Verification items for the finished model (mm, model axes). A direction names the side the tool comes from. Give positions to 0.01 mm unless a question says otherwise; leave off trailing zeros. Write each loop counter-clockwise with the first axis right and the second up, starting at its lowest first coordinate (ties: lowest second). Pieces come first, ordered by that corner, then holes. Notation, with made-up numbers: (-11.5, 9) -> (37.5, 9) arc R23 ccw to (37.5, 27) -> close; hole circle Ø2 at (77.5, 70.5). An arc over 180 degrees is marked (long way). Use one line per item in the form item = value. Start each with the question number.
(1) Section check D-D, the plane y = 6. Record the cut outline in (x, z).
(2) Section check A-A, the plane x = 0.5. Record the cut outline in (y, z).
(3) Set-up check for faces 4 (the face through (-61.486, 1, -29)), 5 (the face through (-23, 2.5, 14)), 6 (the face through (-63.486, 27, 26)), 7 (the face through (-17.486, 1, 26)): record each of +Z, -Z, +X, -X, +Y, -Y from which the full face is reachable in a straight line by a thin tool's end or side.
(4) Section check C-C, the plane z = -5. Record the cut outline in (x, y), plus the area to 3 significant figures.
(5) Scan lines: L1, parallel to X at y = 5.5, z = 20.5; L2, parallel to Z at x = 31, y = 7.25; L3, parallel to Y at x = -4.5, z = 20. Record each from-to range of solid material in increasing order.
(6) Section check B-B, the plane y = 20. State how many separate pieces and enclosed holes the cut face has, plus the area to 4 significant figures.
(7) Depth check by flat-ended pin: pin 1 Ø9.5 at (x, z) = (-23.49, -16.85) entering from +Y; pin 2 Ø1.5 at (y, z) = (28, 25.5) entering from +X; pin 3 Ø3.5 at (y, z) = (16, -29.5) entering from +X. Enter the tip coordinate at first touch or a pass-through.
(8) Release check for a two-part mould opening along Y. For faces 1 (the face through (-64.486, 10, -29)), 2 (the face through (-19, 3, -2)), 3 (the face through (-21.26, 1.23, 11.6)) record: pulls with the +Y half, pulls with the -Y half, needs draft (parallel to the pull), parting line crosses it, or undercut.
from build123d import *

# Parameters (mm, degrees)
SKETCH2_W           = 114
SKETCH2_H           = 58
BOSS_EXTRUDE1_DEPTH = 3
SKETCH3_R           = 1.5
CUT_EXTRUDE5_DEPTH  = 4
SKETCH5_R           = 3.025
CUT_EXTRUDE7_DEPTH  = 2.5
SKETCH7_W           = 3
SKETCH7_H           = 52
BOSS_EXTRUDE2_DEPTH = 22
CUT_EXTRUDE8_REACH  = 5
SKETCH8_R           = 1.5
CUT_EXTRUDE9_REACH  = 60
SKETCH9_W           = 50
SKETCH9_H           = 10
CUT_EXTRUDE10_REACH = 116
SKETCH10_W          = 32
SKETCH10_H          = 6
SKETCH10_W_2        = 12
SKETCH10_H_2        = 8
CUT_EXTRUDE11_REACH = 60
SKETCH11_W          = 70
SKETCH11_H          = 12
SKETCH12_R          = 1.25
CUT_EXTRUDE12_DEPTH = 59
SKETCH13_W          = 13
SKETCH13_H          = 5
BOSS_EXTRUDE4_DEPTH = 3
SKETCH14_W          = 13
SKETCH14_H          = 5
BOSS_EXTRUDE5_DEPTH = 3
SKETCH15_R          = 1.25
CUT_EXTRUDE13_DEPTH = 59
SKETCH16_W          = 2
SKETCH16_H          = 5
BOSS_EXTRUDE6_DEPTH = 3
CUT_EXTRUDE14_REACH = 5
SKETCH17_R          = 3.5
SKETCH19_W          = 1
SKETCH19_H          = 58
BOSS_EXTRUDE7_DEPTH = 9
CUT_EXTRUDE15_REACH = 117
SKETCH20_W          = 28
SKETCH20_H          = 5
SKETCH21_W          = 10
SKETCH21_H          = 2.5
CUT_EXTRUDE16_DEPTH = 2.2


with BuildPart() as part:
    # Sketch2 → Boss-Extrude1 (new body)
    with BuildSketch(Plane(origin=(0, 0, 0), x_dir=(1, 0, 0), z_dir=(0, 1, 0))):
        with Locations((-19.486211897, 1.601935214)):
            Rectangle(SKETCH2_W, SKETCH2_H)
    extrude(amount=BOSS_EXTRUDE1_DEPTH)

    # Sketch3 → Cut-Extrude5 (cut, through all)
    with BuildSketch(Plane(origin=(0, 3, 0), x_dir=(1, 0, 0), z_dir=(0, 1, 0))):
        with Locations((-10.486211897, 13.601935214)):
            Circle(SKETCH3_R)
        with Locations((-10.486211897, -10.398064786)):
            Circle(SKETCH3_R)
        with Locations((-68.986211897, 1.601935214)):
            Circle(SKETCH3_R)
    extrude(amount=-CUT_EXTRUDE5_DEPTH, mode=Mode.SUBTRACT)

    # Sketch5 → Cut-Extrude7 (cut)
    with BuildSketch(Plane(origin=(0, 0, 0), x_dir=(-1, 0, 0), z_dir=(0, -1, 0))):
        with Locations((23.486211897, 16.851935214)):
            Circle(SKETCH5_R)
        with Locations((23.486211897, -13.648064786)):
            Circle(SKETCH5_R)
        with Locations((53.986211897, -13.648064786)):
            Circle(SKETCH5_R)
        with Locations((53.986211897, 16.851935214)):
            Circle(SKETCH5_R)
    extrude(amount=-CUT_EXTRUDE7_DEPTH, mode=Mode.SUBTRACT)

    # Sketch7 → Boss-Extrude2 (add)
    with BuildSketch(Plane(origin=(0, 3, 0), x_dir=(1, 0, 0), z_dir=(0, 1, 0))):
        Polygon((37.513788103, 30.601935214), (-76.486211897, 30.601935214), (-76.486211897, 27.601935214), (-73.486211897, 27.601935214), (37.513788103, 27.601935214), align=None)
        with Locations((-74.986211897, 1.601935214)):
            Rectangle(SKETCH7_W, SKETCH7_H)
        Polygon((-73.486211897, -24.398064786), (-76.486211897, -24.398064786), (-76.486211897, -27.398064786), (37.513788103, -27.398064786), (37.513788103, -24.398064786), align=None)
    extrude(amount=BOSS_EXTRUDE2_DEPTH)

    # Sketch8 → Cut-Extrude8 (cut, up to next)
    with BuildSketch(Plane(origin=(0, 3, 0), x_dir=(1, 0, 0), z_dir=(0, 1, 0)), mode=Mode.PRIVATE) as cut_extrude8_sk1:
        with Locations((-69.486211897, 21.601935214)):
            Circle(SKETCH8_R)
    cut_extrude8_tool1 = extrude(cut_extrude8_sk1.sketch, amount=-CUT_EXTRUDE8_REACH, mode=Mode.PRIVATE) & part.part
    add(cut_extrude8_tool1.solids().sort_by_distance((-69.486212, 3, -21.601935))[0], mode=Mode.SUBTRACT)
    # Sketch8 → Cut-Extrude8 (cut, up to next)
    with BuildSketch(Plane(origin=(0, 3, 0), x_dir=(1, 0, 0), z_dir=(0, 1, 0)), mode=Mode.PRIVATE) as cut_extrude8_sk2:
        with Locations((-69.486211897, -20.398064786)):
            Circle(SKETCH8_R)
    cut_extrude8_tool2 = extrude(cut_extrude8_sk2.sketch, amount=-CUT_EXTRUDE8_REACH, mode=Mode.PRIVATE) & part.part
    add(cut_extrude8_tool2.solids().sort_by_distance((-69.486212, 3, 20.398065))[0], mode=Mode.SUBTRACT)
    # Sketch8 → Cut-Extrude8 (cut, up to next)
    with BuildSketch(Plane(origin=(0, 3, 0), x_dir=(1, 0, 0), z_dir=(0, 1, 0)), mode=Mode.PRIVATE) as cut_extrude8_sk3:
        with Locations((9.513788103, 21.601935214)):
            Circle(SKETCH8_R)
    cut_extrude8_tool3 = extrude(cut_extrude8_sk3.sketch, amount=-CUT_EXTRUDE8_REACH, mode=Mode.PRIVATE) & part.part
    add(cut_extrude8_tool3.solids().sort_by_distance((9.513788, 3, -21.601935))[0], mode=Mode.SUBTRACT)
    # Sketch8 → Cut-Extrude8 (cut, up to next)
    with BuildSketch(Plane(origin=(0, 3, 0), x_dir=(1, 0, 0), z_dir=(0, 1, 0)), mode=Mode.PRIVATE) as cut_extrude8_sk4:
        with Locations((9.513788103, -20.398064786)):
            Circle(SKETCH8_R)
    cut_extrude8_tool4 = extrude(cut_extrude8_sk4.sketch, amount=-CUT_EXTRUDE8_REACH, mode=Mode.PRIVATE) & part.part
    add(cut_extrude8_tool4.solids().sort_by_distance((9.513788, 3, 20.398065))[0], mode=Mode.SUBTRACT)

    # Sketch9 → Cut-Extrude9 (cut, up to next)
    with BuildSketch(Plane.XY.offset(27.398064786), mode=Mode.PRIVATE) as cut_extrude9_sk1:
        with Locations((-29.486211897, 20)):
            Rectangle(SKETCH9_W, SKETCH9_H)
    cut_extrude9_tool1 = extrude(cut_extrude9_sk1.sketch, amount=-CUT_EXTRUDE9_REACH, mode=Mode.PRIVATE) & part.part
    add(cut_extrude9_tool1.solids().sort_by_distance((-29.486212, 20, 27.398065))[0], mode=Mode.SUBTRACT)

    # Sketch10 → Cut-Extrude10 (cut, up to next)
    with BuildSketch(Plane.ZY.offset(76.486211897), mode=Mode.PRIVATE) as cut_extrude10_sk1:
        with Locations((-3.601935214, 7)):
            Rectangle(SKETCH10_W, SKETCH10_H)
    cut_extrude10_tool1 = extrude(cut_extrude10_sk1.sketch, amount=-CUT_EXTRUDE10_REACH, mode=Mode.PRIVATE) & part.part
    add(cut_extrude10_tool1.solids().sort_by_distance((-76.486212, 7, -3.601935))[0], mode=Mode.SUBTRACT)
    # Sketch10 → Cut-Extrude10 (cut, up to next)
    with BuildSketch(Plane.ZY.offset(76.486211897), mode=Mode.PRIVATE) as cut_extrude10_sk2:
        with Locations((-12.601935214, 21)):
            Rectangle(SKETCH10_W_2, SKETCH10_H_2)
    cut_extrude10_tool2 = extrude(cut_extrude10_sk2.sketch, amount=-CUT_EXTRUDE10_REACH, mode=Mode.PRIVATE) & part.part
    add(cut_extrude10_tool2.solids().sort_by_distance((-76.486212, 21, -12.601935))[0], mode=Mode.SUBTRACT)

    # Sketch11 → Cut-Extrude11 (cut, up to next)
    with BuildSketch(Plane(origin=(0, 0, -30.601935214), x_dir=(-1, 0, 0), z_dir=(0, 0, -1)), mode=Mode.PRIVATE) as cut_extrude11_sk1:
        with Locations((29.486211897, 10)):
            Rectangle(SKETCH11_W, SKETCH11_H)
    cut_extrude11_tool1 = extrude(cut_extrude11_sk1.sketch, amount=-CUT_EXTRUDE11_REACH, mode=Mode.PRIVATE) & part.part
    add(cut_extrude11_tool1.solids().sort_by_distance((-29.486212, 10, -30.601935))[0], mode=Mode.SUBTRACT)

    # Sketch12 → Cut-Extrude12 (cut, through all)
    with BuildSketch(Plane.XY.offset(27.398064786)):
        with Locations((22.513788103, 20)):
            Circle(SKETCH12_R)
        with Locations((32.513788103, 20)):
            Circle(SKETCH12_R)
        with Locations((-68.488300827, 11)):
            Circle(SKETCH12_R)
    extrude(amount=-CUT_EXTRUDE12_DEPTH, mode=Mode.SUBTRACT)

    # Sketch13 → Boss-Extrude4 (add)
    with BuildSketch(Plane.XY.offset(27.398064786)):
        with Locations((-69.986211897, 27.5)):
            Rectangle(SKETCH13_W, SKETCH13_H)
    extrude(amount=-BOSS_EXTRUDE4_DEPTH)

    # Sketch14 → Boss-Extrude5 (add)
    with BuildSketch(Plane(origin=(0, 0, -30.601935214), x_dir=(-1, 0, 0), z_dir=(0, 0, -1))):
        with Locations((69.986211897, 27.5)):
            Rectangle(SKETCH14_W, SKETCH14_H)
    extrude(amount=-BOSS_EXTRUDE5_DEPTH)

    # Sketch15 → Cut-Extrude13 (cut, through all)
    with BuildSketch(Plane.XY.offset(27.398064786)):
        with Locations((-68.486211897, 26)):
            Circle(SKETCH15_R)
    extrude(amount=-CUT_EXTRUDE13_DEPTH, mode=Mode.SUBTRACT)

    # Sketch16 → Boss-Extrude6 (add)
    with BuildSketch(Plane.ZY.offset(76.486211897)):
        with Locations((23.398064786, 27.5)):
            Rectangle(SKETCH16_W, SKETCH16_H)
        with Locations((-26.601935214, 27.5)):
            Rectangle(SKETCH16_W, SKETCH16_H)
    extrude(amount=-BOSS_EXTRUDE6_DEPTH)

    # Sketch17 → Cut-Extrude14 (cut, up to next)
    with BuildSketch(Plane.XY.offset(-27.601935214), mode=Mode.PRIVATE) as cut_extrude14_sk1:
        with Locations((22.513788103, 20)):
            Circle(SKETCH17_R)
    cut_extrude14_tool1 = extrude(cut_extrude14_sk1.sketch, amount=-CUT_EXTRUDE14_REACH, mode=Mode.PRIVATE) & part.part
    add(cut_extrude14_tool1.solids().sort_by_distance((22.513788, 20, -27.601935))[0], mode=Mode.SUBTRACT)

    # Sketch19 → Boss-Extrude7 (add)
    with BuildSketch(Plane.XZ):
        with Locations((38.013788103, -1.601935214)):
            Rectangle(SKETCH19_W, SKETCH19_H)
    extrude(amount=-BOSS_EXTRUDE7_DEPTH)

    # Sketch20 → Cut-Extrude15 (cut, up to next)
    with BuildSketch(Plane(origin=(38.513788103, 0, 0), x_dir=(0, 0, -1), z_dir=(1, 0, 0)), mode=Mode.PRIVATE) as cut_extrude15_sk1:
        with Locations((-4.398064786, 6.5)):
            Rectangle(SKETCH20_W, SKETCH20_H)
    cut_extrude15_tool1 = extrude(cut_extrude15_sk1.sketch, amount=-CUT_EXTRUDE15_REACH, mode=Mode.PRIVATE) & part.part
    add(cut_extrude15_tool1.solids().sort_by_distance((38.513788, 6.5, 4.398065))[0], mode=Mode.SUBTRACT)

    # Sketch21 → Cut-Extrude16 (cut)
    with BuildSketch(Plane(origin=(0, 0, 0), x_dir=(-1, 0, 0), z_dir=(0, -1, 0))):
        with Locations((66.486211897, -26.148064786)):
            Rectangle(SKETCH21_W, SKETCH21_H)
        with Locations((12.486211897, -26.148064786)):
            Rectangle(SKETCH21_W, SKETCH21_H)
        with Locations((12.486211897, 29.351935214)):
            Rectangle(SKETCH21_W, SKETCH21_H)
        with Locations((66.486211897, 29.351935214)):
            Rectangle(SKETCH21_W, SKETCH21_H)
    extrude(amount=-CUT_EXTRUDE16_DEPTH, mode=Mode.SUBTRACT)


solid = part.part
Completed:
q1.outline = (-76.49, -30.6) -> (-64.49, -30.6) -> (-64.49, -27.6) -> (-73.49, -27.6) -> (-73.49, -19.6) -> (-76.49, -19.6) -> close; (-76.49, 12.4) -> (-73.49, 12.4) -> (-73.49, 24.4) -> (37.51, 24.4) -> (37.51, 18.4) -> (38.51, 18.4) -> (38.51, 27.4) -> (-76.49, 27.4) -> close; (5.51, -30.6) -> (38.51, -30.6) -> (38.51, -9.6) -> (37.51, -9.6) -> (37.51, -27.6) -> (5.51, -27.6) -> close
q2.outline = (0, -30.6) -> (4, -30.6) -> (4, -27.6) -> (3, -27.6) -> (3, 24.4) -> (25, 24.4) -> (25, 27.4) -> (0, 27.4) -> close; (16, -30.6) -> (25, -30.6) -> (25, -27.6) -> (16, -27.6) -> close
q3.face_4 = -Z, -Y
q3.face_5 = -Y
q3.face_6 = +Z, -Z, +X, +Y
q3.face_7 = +Z, -Y
q4.outline = (-76.49, 0) -> (38.51, 0) -> (38.51, 4) -> (37.51, 4) -> (37.51, 3) -> (-73.49, 3) -> (-73.49, 4) -> (-76.49, 4) -> close; (-76.49, 10) -> (-73.49, 10) -> (-73.49, 25) -> (-76.49, 25) -> close
q4.area = 394 mm²
q5.L1 = -76.49 to -73.49, 37.51 to 38.51
q5.L2 = -30.6 to -27.6, 24.4 to 27.4
q5.L3 = 0 to 3
q6.separate_pieces = 7
q6.enclosed_holes = 0
q6.area = 610.5 mm²
q7.pin_1 = 3
q7.pin_2 = -63.49
q7.pin_3 = 37.51
q8.face_1 = undercut
q8.face_2 = pulls with the +Y half
q8.face_3 = needs draft
